Source: CAD feature listing. Evaluate the final solid. Frame: model axes, mm. Face numbers are marked on the shaded views. Coordinates: 2 decimals unless noted, no trailing zeros. Loops run counter-clockwise (first coordinate to the right, second up) from the corner with the lowest first, then second, coordinate; pieces in that order, holes last.
```python
from build123d import *

# Parameters (mm, degrees)
BOSS_EXTRUDE2_DEPTH = 15
SKETCH4_R           = 2.5
CUT_EXTRUDE1_DEPTH  = 15
SKETCH5_R           = 4.25
CUT_EXTRUDE6_DEPTH  = 5
SKETCH6_W           = 5
SKETCH6_H           = 2
CUT_EXTRUDE7_DEPTH  = 43.267768571
FILLET1_R           = 1


with BuildPart() as part:
    # Sketch2 → Boss-Extrude2 (new body)
    with BuildSketch(Plane.XY):
        with BuildLine():
            Line((0, 15), (0, 0))
            Line((0, 0), (36.559051501, 0))
            Line((36.559051501, 0), (36.559051501, 15))
            ThreePointArc((36.559051501, 15), (18.27952575, 9.847260148), (0, 15))
        make_face()
    extrude(amount=BOSS_EXTRUDE2_DEPTH)

    # Sketch4 → Cut-Extrude1 (cut)
    with BuildSketch(Plane.XZ):
        with Locations(Location((22.559051501, 7.5, 0), (0, 0, 270))):
            Circle(SKETCH4_R)
    extrude(amount=-CUT_EXTRUDE1_DEPTH, mode=Mode.SUBTRACT)

    # Sketch5 → Cut-Extrude6 (cut, symmetric)
    with BuildSketch(Plane(origin=(0, 9.847260148, 0), x_dir=(1, 0, 0), z_dir=(0, 1, 0))):
        with Locations(Location((22.559051501, -7.5, 0), (0, 0, 270))):
            Circle(SKETCH5_R)
    extrude(amount=CUT_EXTRUDE6_DEPTH, both=True, mode=Mode.SUBTRACT)

    # Sketch6 → Cut-Extrude7 (cut, through all)
    with BuildSketch(Plane(origin=(36.559051501, 0, 0), x_dir=(0, 0, -1), z_dir=(1, 0, 0))):
        with Locations((-3.5, 7.5)):
            Rectangle(SKETCH6_W, SKETCH6_H)
    extrude(amount=-CUT_EXTRUDE7_DEPTH, mode=Mode.SUBTRACT)

    # Fillet1
    fillet1_edges = [part.edges().sort_by_distance(p)[0] for p in [
        (0, 15, 7.5),
        (36.559051501, 15, 7.5),
    ]]
    fillet(fillet1_edges, radius=FILLET1_R)


solid = part.part
```
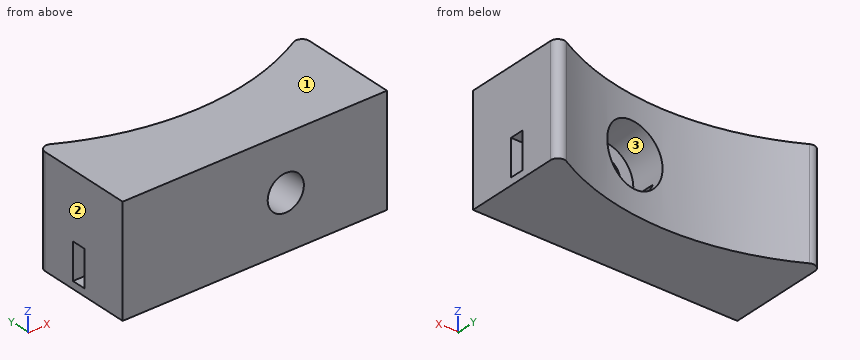
Q1. Section query D-D on x = 8. Return the cut outline in (y, z), then the cut area to 3 significant figures.
Q2. Section query A-A on z = 7.5. Return the cut outline in (x, y).
Q3. Draft query along Z for the marked faces 1, 2 and 3. Return one class per face: released by +Z, released by -Z, zero draft, split by the parting line, or undercut.
Q4. Section query B-B on x = 32. Return the cut outline in (y, z), then the cut area to 3 significant figures.
Q5. Section query C-C on y = 2. Return the cut outline in (x, z).
Q6. Material intervals for line 1 along X through (y, z) = (2.1, 7.5); line 2 along X through (y, z) = (6.25, 7.5); line 3 along Z through (x, y) = (12, 8.25), sorted ascending.
Q7. First-contact query: pin 1 Ø2 at (x, y) = (8, 8) entering from -Z; pin 2 Ø5.5 at (x, z) = (19, 3) entering from +Y; pin 3 Ø8 at (x, z) = (22.56, 7.5) entering from +Y; pin 4 Ø1 at (x, z) = (23, 11.5) entering from +Y. Flat tips, straight axial feed; report the tip coordinate or a pass-through.
Resolved:
1. outline: (0, 0) - (11.39, 0) - (11.39, 15) - (0, 15) - close; hole (6.5, 1) - (8.5, 1) - (8.5, 6) - (6.5, 6) - close
1. area: 161 mm2
2. outline: (0, 0) - (20.06, 0) - (20.06, 4.85) - (18.31, 4.85) - (18.31, 9.85) arc R35 cw to (1.48, 14.14) arc R1 ccw to (0, 13.27) - close; (25.06, 0) - (36.56, 0) - (36.56, 13.27) arc R1 ccw to (35.08, 14.14) arc R35 cw to (26.81, 10.9) - (26.81, 4.85) - (25.06, 4.85) - close
3. face 1: released by +Z
3. face 2: zero draft
3. face 3: undercut
4. outline: (0, 0) - (12.65, 0) - (12.65, 15) - (0, 15) - close; hole (6.5, 1) - (8.5, 1) - (8.5, 6) - (6.5, 6) - close
4. area: 180 mm2
5. outline: (0, 0) - (36.56, 0) - (36.56, 15) - (0, 15) - close; hole circle Ø5 at (22.56, 7.5)
6. line 1: x = 0 to 20.06, 25.06 to 36.56
6. line 2: x = 0 to 18.31, 26.81 to 36.56
6. line 3: z = 0 to 1, 6 to 15
7. pin 1: stops at z = 0
7. pin 2: stops at y = 10.02
7. pin 3: stops at y = 4.85
7. pin 4: stops at y = 10.24
